from build123d import *

# Parameters (mm, degrees)
F0_R     = 27
F1_DEPTH = 1
F2_DEPTH = 8
F3_R     = 1


with BuildPart() as f1:
    # F0 (on Front) → F1 (new body, symmetric)
    with BuildSketch(Plane.XZ):
        with BuildLine():
            ThreePointArc((3.6158782374, 31.2779090152), (0, 28.75), (-3.6158782374, 31.2779090152))
            Line((-3.6158782374, 31.2779090152), (-5.4734823617, 34.5852409081))
            ThreePointArc((-5.4734823617, 34.5852409081), (-5.9827680833, 34.5531193631), (-6.4918656711, 34.5181424295))
            Line((-6.4918656711, 34.5181424295), (-7.2118194024, 34.3749347284))
            ThreePointArc((-7.2118194024, 34.3749347284), (-7.6955493369, 34.2124259891), (-8.1783603743, 34.0472072192))
            Line((-8.1783603743, 34.0472072192), (-8.6289016835, 30.2807566538))
            ThreePointArc((-8.6289016835, 30.2807566538), (-11.0021486805, 26.5615365597), (-15.3101734747, 27.513283264))
            Line((-15.3101734747, 27.513283264), (-18.2920370254, 29.8579851848))
            ThreePointArc((-18.2920370254, 29.8579851848), (-18.7502632967, 29.6334135388), (-19.2072230452, 29.4062758535))
            Line((-19.2072230452, 29.4062758535), (-19.8175703473, 28.9984548245))
            ThreePointArc((-19.8175703473, 28.9984548245), (-20.2022891308, 28.6632008947), (-20.5851218804, 28.3257948698))
            Line((-20.5851218804, 28.3257948698), (-19.5600095444, 24.6736335876))
            ThreePointArc((-19.5600095444, 24.6736335876), (-20.3293199591, 20.3293199591), (-24.6736335876, 19.5600095444))
            Line((-24.6736335876, 19.5600095444), (-28.3257948698, 20.5851218804))
            ThreePointArc((-28.3257948698, 20.5851218804), (-28.6632008947, 20.2022891308), (-28.9984548245, 19.8175703473))
            Line((-28.9984548245, 19.8175703473), (-29.4062758535, 19.2072230452))
            ThreePointArc((-29.4062758535, 19.2072230452), (-29.6334135388, 18.7502632967), (-29.8579851848, 18.2920370254))
            Line((-29.8579851848, 18.2920370254), (-27.513283264, 15.3101734747))
            ThreePointArc((-27.513283264, 15.3101734747), (-26.5615365597, 11.0021486805), (-30.2807566538, 8.6289016835))
            Line((-30.2807566538, 8.6289016835), (-34.0472072192, 8.1783603743))
            ThreePointArc((-34.0472072192, 8.1783603743), (-34.2124259891, 7.6955493369), (-34.3749347284, 7.2118194024))
            Line((-34.3749347284, 7.2118194024), (-34.5181424295, 6.4918656711))
            ThreePointArc((-34.5181424295, 6.4918656711), (-34.5531193631, 5.9827680833), (-34.5852409081, 5.4734823617))
            Line((-34.5852409081, 5.4734823617), (-31.2779090152, 3.6158782374))
            ThreePointArc((-31.2779090152, 3.6158782374), (-28.75, 0), (-31.2779090152, -3.6158782374))
            Line((-31.2779090152, -3.6158782374), (-34.5852409081, -5.4734823617))
            ThreePointArc((-34.5852409081, -5.4734823617), (-34.5531193631, -5.9827680833), (-34.5181424295, -6.4918656711))
            Line((-34.5181424295, -6.4918656711), (-34.3749347284, -7.2118194024))
            ThreePointArc((-34.3749347284, -7.2118194024), (-34.2124259891, -7.6955493369), (-34.0472072192, -8.1783603743))
            Line((-34.0472072192, -8.1783603743), (-30.2807566538, -8.6289016835))
            ThreePointArc((-30.2807566538, -8.6289016835), (-26.5615365597, -11.0021486805), (-27.513283264, -15.3101734747))
            Line((-27.513283264, -15.3101734747), (-29.8579851848, -18.2920370254))
            ThreePointArc((-29.8579851848, -18.2920370254), (-29.6334135388, -18.7502632967), (-29.4062758535, -19.2072230452))
            Line((-29.4062758535, -19.2072230452), (-28.9984548245, -19.8175703473))
            ThreePointArc((-28.9984548245, -19.8175703473), (-28.6632008947, -20.2022891308), (-28.3257948698, -20.5851218804))
            Line((-28.3257948698, -20.5851218804), (-24.6736335876, -19.5600095444))
            ThreePointArc((-24.6736335876, -19.5600095444), (-20.3293199591, -20.3293199591), (-19.5600095444, -24.6736335876))
            Line((-19.5600095444, -24.6736335876), (-20.5851218804, -28.3257948698))
            ThreePointArc((-20.5851218804, -28.3257948698), (-20.2022891308, -28.6632008947), (-19.8175703473, -28.9984548245))
            Line((-19.8175703473, -28.9984548245), (-19.2072230452, -29.4062758535))
            ThreePointArc((-19.2072230452, -29.4062758535), (-18.7502632967, -29.6334135388), (-18.2920370254, -29.8579851848))
            Line((-18.2920370254, -29.8579851848), (-15.3101734747, -27.513283264))
            ThreePointArc((-15.3101734747, -27.513283264), (-11.0021486805, -26.5615365597), (-8.6289016835, -30.2807566538))
            Line((-8.6289016835, -30.2807566538), (-8.1783603743, -34.0472072192))
            ThreePointArc((-8.1783603743, -34.0472072192), (-7.6955493369, -34.2124259891), (-7.2118194024, -34.3749347284))
            Line((-7.2118194024, -34.3749347284), (-6.4918656711, -34.5181424295))
            ThreePointArc((-6.4918656711, -34.5181424295), (-5.9827680833, -34.5531193631), (-5.4734823617, -34.5852409081))
            Line((-5.4734823617, -34.5852409081), (-3.6158782374, -31.2779090152))
            ThreePointArc((-3.6158782374, -31.2779090152), (0, -28.75), (3.6158782374, -31.2779090152))
            Line((3.6158782374, -31.2779090152), (5.4734823617, -34.5852409081))
            ThreePointArc((5.4734823617, -34.5852409081), (5.9827680833, -34.5531193631), (6.4918656711, -34.5181424295))
            Line((6.4918656711, -34.5181424295), (7.2118194024, -34.3749347284))
            ThreePointArc((7.2118194024, -34.3749347284), (7.6955493369, -34.2124259891), (8.1783603743, -34.0472072192))
            Line((8.1783603743, -34.0472072192), (8.6289016835, -30.2807566538))
            ThreePointArc((8.6289016835, -30.2807566538), (11.0021486805, -26.5615365597), (15.3101734747, -27.513283264))
            Line((15.3101734747, -27.513283264), (18.2920370254, -29.8579851848))
            ThreePointArc((18.2920370254, -29.8579851848), (18.7502632967, -29.6334135388), (19.2072230452, -29.4062758535))
            Line((19.2072230452, -29.4062758535), (19.8175703473, -28.9984548245))
            ThreePointArc((19.8175703473, -28.9984548245), (20.2022891308, -28.6632008947), (20.5851218804, -28.3257948698))
            Line((20.5851218804, -28.3257948698), (19.5600095444, -24.6736335876))
            ThreePointArc((19.5600095444, -24.6736335876), (20.3293199591, -20.3293199591), (24.6736335876, -19.5600095444))
            Line((24.6736335876, -19.5600095444), (28.3257948698, -20.5851218804))
            ThreePointArc((28.3257948698, -20.5851218804), (28.6632008947, -20.2022891308), (28.9984548245, -19.8175703473))
            Line((28.9984548245, -19.8175703473), (29.4062758535, -19.2072230452))
            ThreePointArc((29.4062758535, -19.2072230452), (29.6334135388, -18.7502632967), (29.8579851848, -18.2920370254))
            Line((29.8579851848, -18.2920370254), (27.513283264, -15.3101734747))
            ThreePointArc((27.513283264, -15.3101734747), (26.5615365597, -11.0021486805), (30.2807566538, -8.6289016835))
            Line((30.2807566538, -8.6289016835), (34.0472072192, -8.1783603743))
            ThreePointArc((34.0472072192, -8.1783603743), (34.2124259891, -7.6955493369), (34.3749347284, -7.2118194024))
            Line((34.3749347284, -7.2118194024), (34.5181424295, -6.4918656711))
            ThreePointArc((34.5181424295, -6.4918656711), (34.5531193631, -5.9827680833), (34.5852409081, -5.4734823617))
            Line((34.5852409081, -5.4734823617), (31.2779090152, -3.6158782374))
            ThreePointArc((31.2779090152, -3.6158782374), (28.75, 0), (31.2779090152, 3.6158782374))
            Line((31.2779090152, 3.6158782374), (34.5852409081, 5.4734823617))
            ThreePointArc((34.5852409081, 5.4734823617), (34.5531193631, 5.9827680833), (34.5181424295, 6.4918656711))
            Line((34.5181424295, 6.4918656711), (34.3749347284, 7.2118194024))
            ThreePointArc((34.3749347284, 7.2118194024), (34.2124259891, 7.6955493369), (34.0472072192, 8.1783603743))
            Line((34.0472072192, 8.1783603743), (30.2807566538, 8.6289016835))
            ThreePointArc((30.2807566538, 8.6289016835), (26.5615365597, 11.0021486805), (27.513283264, 15.3101734747))
            Line((27.513283264, 15.3101734747), (29.8579851848, 18.2920370254))
            ThreePointArc((29.8579851848, 18.2920370254), (29.6334135388, 18.7502632967), (29.4062758535, 19.2072230452))
            Line((29.4062758535, 19.2072230452), (28.9984548245, 19.8175703473))
            ThreePointArc((28.9984548245, 19.8175703473), (28.6632008947, 20.2022891308), (28.3257948698, 20.5851218804))
            Line((28.3257948698, 20.5851218804), (24.6736335876, 19.5600095444))
            ThreePointArc((24.6736335876, 19.5600095444), (20.3293199591, 20.3293199591), (19.5600095444, 24.6736335876))
            Line((19.5600095444, 24.6736335876), (20.5851218804, 28.3257948698))
            ThreePointArc((20.5851218804, 28.3257948698), (20.2022891308, 28.6632008947), (19.8175703473, 28.9984548245))
            Line((19.8175703473, 28.9984548245), (19.2072230452, 29.4062758535))
            ThreePointArc((19.2072230452, 29.4062758535), (18.7502632967, 29.6334135388), (18.2920370254, 29.8579851848))
            Line((18.2920370254, 29.8579851848), (15.3101734747, 27.513283264))
            ThreePointArc((15.3101734747, 27.513283264), (11.0021486805, 26.5615365597), (8.6289016835, 30.2807566538))
            Line((8.6289016835, 30.2807566538), (8.1783603743, 34.0472072192))
            ThreePointArc((8.1783603743, 34.0472072192), (7.6955493369, 34.2124259891), (7.2118194024, 34.3749347284))
            Line((7.2118194024, 34.3749347284), (6.4918656711, 34.5181424295))
            ThreePointArc((6.4918656711, 34.5181424295), (5.9827680833, 34.5531193631), (5.4734823617, 34.5852409081))
            Line((5.4734823617, 34.5852409081), (3.6158782374, 31.2779090152))
        make_face()
        Circle(F0_R, mode=Mode.SUBTRACT)
    extrude(amount=F1_DEPTH, both=True)

    # F0 (on Front) → F2 (join, symmetric)
    with BuildSketch(Plane.XZ):
        Circle(F0_R)
    extrude(amount=F2_DEPTH, both=True)

    # F3
    f3_edges = [f1.edges().sort_by_distance(p)[0] for p in [
        (-27, -8, 0),
        (-27, 8, 0),
    ]]
    fillet(f3_edges, radius=F3_R)


solid = f1.part
Could you check a few things on this model? Use its own coordinates, in mm. A direction names the side the tool comes from. Coordinates: 2 decimals unless noted, no trailing zeros. Order: outer loops, then holes, each group sorted by start corner. A loop starts at its lowest first (then second) coordinate and runs counter-clockwise, first axis right, second up.
Q1. Will these pins go through, and if not, where does the flat tip stop? pin 1 (2 mm diameter, centred on y = -0.5, z = -3, fed in from -X); pin 2 (3 mm diameter, centred on y = 5.5, z = 10, fed in from +X); pin 3 (8 mm diameter, centred on x = 3.5, y = 6, fed in from -Z).
Q2. Suppose I cut it at B-B on z = 0. Please give me the cut outline in (x, y).
Q3. Please list where these lines run through material, in increasing order: L1, parallel to Y at x = 7.5, z = -27.5; L2, parallel to X at y = 0.25, z = 3; L3, parallel to X at y = 5.5, z = 1.5.
Q4. Suppose I cut it at C-C on y = 4. Please give me the cut outline in (x, z).
Q5. Which directions (+Z, -Z, +X, -X, +Y, -Y) give clear straight access to the entire face, cutting with the end or side of a thin tool? Please do faces 4 (the flat face through (28.67, -0.01, 16.78)), 5 (the flat face through (-28.67, -0.01, -16.78)), 6 (the flat face through (-4.558, -0.014, -32.955)).
Q6. Suppose I cut it at A-A on x = 0. Please give me the cut outline in (y, z).
Q7. Thinking about a two-plate mould opening in Z: for faces 1 (the flat face through (32.908, -0.014, 4.532)), 2 (the flat face through (32.2, 0, 8.4)), 3 (the flat face through (-16.82, -0.01, -28.7)), which applies, released by +Z, released by -Z, zero draft, split by the parting line, or undercut?
Answer:
1. pin 1: stops at x = -31.96
1. pin 2: stops at x = 25.63
1. pin 3: stops at z = -27
2. outline: (-28.75, -1) - (-27, -1) - (-27, -7) arc R1 ccw to (-26, -8) - (26, -8) arc R1 ccw to (27, -7) - (27, -1) - (28.75, -1) - (28.75, 1) - (27, 1) - (27, 7) arc R1 ccw to (26, 8) - (-26, 8) arc R1 ccw to (-27, 7) - (-27, 1) - (-28.75, 1) - close
3. L1: y = -1 to 1
3. L2: x = -30.19 to 30.19
3. L3: x = -26.96 to 26.96
4. outline: circle Ø54 at (0, 0)
5. face 4: +X, +Y, -Y
5. face 5: -X, +Y, -Y
5. face 6: -Z, +Y, -Y
6. outline: (-8, -26) arc R1 ccw to (-7, -27) - (-1, -27) - (-1, -28.75) - (1, -28.75) - (1, -27) - (7, -27) arc R1 ccw to (8, -26) - (8, 26) arc R1 ccw to (7, 27) - (1, 27) - (1, 28.75) - (-1, 28.75) - (-1, 27) - (-7, 27) arc R1 ccw to (-8, 26) - close
7. face 1: undercut
7. face 2: released by +Z
7. face 3: released by -Z
